Read the model definition and answer for the solid it produces. Units are mm, in the model's axes. Face numbers are marked on the shaded views. A direction names the side the tool comes from. Round coordinates to 2 decimals unless told otherwise and drop trailing zeros. Loops run counter-clockwise (first coordinate to the right, second up) from the corner with the lowest first, then second, coordinate; pieces in that order, holes last. Notation, with made-up numbers: (7.5, 1) -> (11.5, 1) arc R5 ccw to (11.5, 8) -> close; hole circle Ø6 at (61, -38.75). An arc over 180 degrees is marked (long way). Put each result on its own line as item: value.
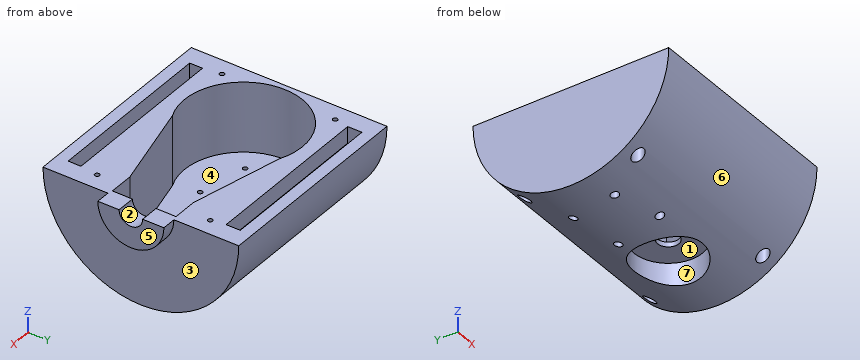
from build123d import *

# Parameters (mm, degrees)
BOSS_EXTRUDE2_DEPTH = 87
CUT_EXTRUDE1_DEPTH  = 29.5
SKETCH3_R           = 4.5
SKETCH3_R_2         = 1
CUT_EXTRUDE2_DEPTH  = 130.771336418
SKETCH4_R           = 14.5
SKETCH4_R_2         = 1.7
CUT_EXTRUDE3_DEPTH  = 10
BOSS_EXTRUDE3_START = 2
BOSS_EXTRUDE3_DEPTH = 2
BOSS_EXTRUDE4_START = 6
BOSS_EXTRUDE4_DEPTH = 6
SKETCH7_W           = 73
SKETCH7_H           = 6
SKETCH7_H_2         = 5.446782016
CUT_EXTRUDE4_DEPTH  = 7
SKETCH8_R           = 1
CUT_EXTRUDE5_DEPTH  = 136.438914135
SKETCH9_R           = 2.5
CUT_EXTRUDE6_DEPTH  = 32


with BuildPart() as part:
    # Sketch1 → Boss-Extrude2 (new body)
    with BuildSketch(Plane(origin=(89.94373008, 0, 0), x_dir=(0, 0, -1), z_dir=(1, 0, 0))):
        with BuildLine():
            Line((-104.016306216, 83.836001664), (-104.016306216, 0.836001664))
            ThreePointArc((-104.016306216, 0.836001664), (-62.516306216, 42.336001664), (-104.016306216, 83.836001664))
        make_face()
    extrude(amount=-BOSS_EXTRUDE2_DEPTH)

    # Sketch2 → Cut-Extrude1 (cut)
    with BuildSketch(Plane.XY.offset(104.016306216)):
        with BuildLine():
            Line((89.94373008, 55.836001595), (79.445092487, 55.836001664))
            Line((79.445092487, 55.836001664), (40.551337791, 64.805487997))
            ThreePointArc((40.551337791, 64.805487997), (5.067466824, 42.109927869), (40.551337791, 19.414367741))
            Line((40.551337791, 19.414367741), (79.445092487, 28.836001664))
            Line((79.445092487, 28.836001664), (89.94373008, 28.836001664))
            Line((89.94373008, 28.836001664), (89.94373008, 55.836001595))
        make_face()
    extrude(amount=-CUT_EXTRUDE1_DEPTH, mode=Mode.SUBTRACT)

    # Sketch3 → Cut-Extrude2 (cut, through all)
    with BuildSketch(Plane(origin=(0, 0, 62.516306216), x_dir=(-1, 0, 0), z_dir=(0, 0, -1))):
        with Locations(Location((-61.067466824, 42.109927869, 0), (0, 0, 90))):
            Circle(SKETCH3_R)
        with Locations(Location((-42.657418818, 50.264258545, 0), (0, 0, 90))):
            Circle(SKETCH3_R_2)
        with Locations(Location((-21.913136148, 54.699879864, 0), (0, 0, 90))):
            Circle(SKETCH3_R_2)
        with Locations(Location((-38.2217975, 29.519975875, 0), (0, 0, 90))):
            Circle(SKETCH3_R_2)
        with Locations(Location((-17.477514829, 33.955597193, 0), (0, 0, 90))):
            Circle(SKETCH3_R_2)
    extrude(amount=-CUT_EXTRUDE2_DEPTH, mode=Mode.SUBTRACT)

    # Sketch4 → Cut-Extrude3 (cut)
    with BuildSketch(Plane(origin=(0, 0, 62.516306216), x_dir=(-1, 0, 0), z_dir=(0, 0, -1))):
        with Locations(Location((-61.067466824, 42.109927869, 0), (0, 0, 90))):
            Circle(SKETCH4_R)
        with Locations(Location((-42.657418818, 50.264258545, 0), (0, 0, 90))):
            Circle(SKETCH4_R_2)
        with Locations(Location((-21.913136148, 54.699879864, 0), (0, 0, 90))):
            Circle(SKETCH4_R_2)
        with Locations(Location((-38.2217975, 29.519975875, 0), (0, 0, 90))):
            Circle(SKETCH4_R_2)
        with Locations(Location((-17.477514829, 33.955597193, 0), (0, 0, 90))):
            Circle(SKETCH4_R_2)
    extrude(amount=-CUT_EXTRUDE3_DEPTH, mode=Mode.SUBTRACT)

    # Sketch5 → Boss-Extrude3 (add)
    with BuildSketch(Plane(origin=(89.94373008, 0, 0), x_dir=(0, 0, -1), z_dir=(1, 0, 0)).offset(BOSS_EXTRUDE3_START)):
        with BuildLine():
            Line((-104.016306216, 55.836001595), (-104.016306216, 47.336001664))
            ThreePointArc((-104.016306216, 47.336001664), (-99.016306216, 42.336001664), (-104.016306216, 37.336001664))
            Line((-104.016306216, 37.336001664), (-104.016306216, 28.836001664))
            Line((-104.016306216, 28.836001664), (-104.016306216, 0.836001664))
            ThreePointArc((-104.016306216, 0.836001664), (-62.516306216, 42.336001664), (-104.016306216, 83.836001664))
            Line((-104.016306216, 83.836001664), (-104.016306216, 55.836001595))
        make_face()
    extrude(amount=-BOSS_EXTRUDE3_DEPTH)

    # Sketch6 → Boss-Extrude4 (add)
    with BuildSketch(Plane(origin=(91.94373008, 0, 0), x_dir=(0, 0, -1), z_dir=(1, 0, 0)).offset(BOSS_EXTRUDE4_START)):
        with BuildLine():
            Line((-104.016306216, 56.336001664), (-104.016306216, 47.336001664))
            ThreePointArc((-104.016306216, 47.336001664), (-99.016306216, 42.336001664), (-104.016306216, 37.336001664))
            Line((-104.016306216, 37.336001664), (-104.016306216, 28.336001664))
            ThreePointArc((-104.016306216, 28.336001664), (-90.016306216, 42.336001664), (-104.016306216, 56.336001664))
        make_face()
    extrude(amount=-BOSS_EXTRUDE4_DEPTH)

    # Sketch7 → Cut-Extrude4 (cut)
    with BuildSketch(Plane.XY.offset(104.016306216)):
        with Locations((47.44373008, 75.836001664)):
            Rectangle(SKETCH7_W, SKETCH7_H)
        with Locations((47.44373008, 8.559392672)):
            Rectangle(SKETCH7_W, SKETCH7_H_2)
    extrude(amount=-CUT_EXTRUDE4_DEPTH, mode=Mode.SUBTRACT)

    # Sketch8 → Cut-Extrude5 (cut, through all)
    with BuildSketch(Plane(origin=(0, 0, 62.516306216), x_dir=(-1, 0, 0), z_dir=(0, 0, -1))):
        with Locations(Location((-84.94373008, 66.836001664, 0), (0, 0, 90))):
            Circle(SKETCH8_R)
        with Locations(Location((-84.94373008, 18.836001664, 0), (0, 0, 90))):
            Circle(SKETCH8_R)
        with Locations(Location((-9.94373008, 66.836001664, 0), (0, 0, 90))):
            Circle(SKETCH8_R)
        with Locations(Location((-9.94373008, 18.836001664, 0), (0, 0, 90))):
            Circle(SKETCH8_R)
    extrude(amount=-CUT_EXTRUDE5_DEPTH, mode=Mode.SUBTRACT)

    # Sketch9 → Cut-Extrude6 (cut)
    with BuildSketch(Plane(origin=(0, 0, 62.516306216), x_dir=(-1, 0, 0), z_dir=(0, 0, -1))):
        with Locations(Location((-84.94373008, 66.836001664, 0), (0, 0, 90))):
            Circle(SKETCH9_R)
        with Locations(Location((-84.94373008, 18.836001664, 0), (0, 0, 90))):
            Circle(SKETCH9_R)
        with Locations(Location((-9.94373008, 66.836001664, 0), (0, 0, 90))):
            Circle(SKETCH9_R)
        with Locations(Location((-9.94373008, 18.836001664, 0), (0, 0, 90))):
            Circle(SKETCH9_R)
    extrude(amount=-CUT_EXTRUDE6_DEPTH, mode=Mode.SUBTRACT)


solid = part.part
Item 1: The part is cut by section A-A (z = 88). Determine the outline of the cut face in (x, y), then the cut area to 3 significant figures.
Derived:
outline: (2.94, 4.05) -> (91.94, 4.05) -> (91.94, 80.62) -> (2.94, 80.62) -> close; hole circle Ø5 at (9.94, 18.84); hole circle Ø5 at (9.94, 66.84); hole (40.55, 19.41) -> (79.45, 28.84) -> (89.94, 28.84) -> (89.94, 55.84) -> (79.45, 55.84) -> (40.55, 64.81) arc R25 ccw (long way) to start; hole circle Ø5 at (84.94, 18.84); hole circle Ø5 at (84.94, 66.84)
area: 3,550 mm^2
Item 2: Which of the six approach directions +Z, -Z, +X, -X, +Y, -Y give full straight-line access (tool end or side, diameter ignored) to the marked faces 1, 2, 3 and 4?
Derived:
face 1: -Z
face 2: +Z, +X
face 3: -Z, +X
face 4: +Z
Item 3: The part is cut by section C-C (x = 63.5). Determine the outline of the cut face in (y, z), then the cut area to 3 significant figures.
Derived:
outline: (0.84, 104.02) arc R41.5 ccw to (27.82, 65.14) -> (27.82, 72.52) -> (38.32, 72.52) -> (38.32, 74.52) -> (24.97, 74.52) -> (24.97, 104.02) -> (11.28, 104.02) -> (11.28, 97.02) -> (5.84, 97.02) -> (5.84, 104.02) -> close; (45.9, 72.52) -> (56.4, 72.52) -> (56.4, 64.97) arc R41.5 ccw to (83.84, 104.02) -> (78.84, 104.02) -> (78.84, 97.02) -> (72.84, 97.02) -> (72.84, 104.02) -> (59.51, 104.02) -> (59.51, 74.52) -> (45.9, 74.52) -> close
area: 1,330 mm^2
Item 4: For a pull along Y with two mould halves and no side action, classify the marked faces 5, 6 and 7 as pulls with the +Y half, pulls with the -Y half, needs draft (parallel to the pull), parting line crosses it, or undercut.
Derived:
face 5: needs draft
face 6: parting line crosses it
face 7: undercut
Item 5: Flat-ended cylindrical pins translate along their axes: pin 1 Ø2 at (x, z) = (72, 79.5) entering from -Y; pin 2 Ø10 at (x, y) = (54.5, 38.5) entering from -Z; pin 3 Ø4 at (x, y) = (42.66, 50.26) entering from -Z. Find the tip coordinate at first contact, or state that the pin passes through.
Derived:
pin 1: stops at y = 8.14
pin 2: stops at z = 72.52
pin 3: stops at z = 62.94
Item 6: The part is cut by section D-D (x = 74.5). Determine the outline of the cut face in (y, z).
Derived:
outline: (0.84, 104.02) arc R41.5 ccw to (36.65, 62.91) -> (36.65, 72.52) -> (47.57, 72.52) -> (47.57, 62.85) arc R41.5 ccw to (83.84, 104.02) -> (78.84, 104.02) -> (78.84, 97.02) -> (72.84, 97.02) -> (72.84, 104.02) -> (56.98, 104.02) -> (56.98, 74.52) -> (27.64, 74.52) -> (27.64, 104.02) -> (11.28, 104.02) -> (11.28, 97.02) -> (5.84, 97.02) -> (5.84, 104.02) -> close
Item 7: The part is cut by section B-B (y = 45). Determine the outline of the cut face in (x, z).
Derived:
outline: (2.94, 62.6) -> (46.86, 62.6) -> (46.86, 72.52) -> (57.62, 72.52) -> (57.62, 74.52) -> (5.24, 74.52) -> (5.24, 104.02) -> (2.94, 104.02) -> close; (64.52, 72.52) -> (75.28, 72.52) -> (75.28, 62.6) -> (91.94, 62.6) -> (91.94, 90.27) -> (97.94, 90.27) -> (97.94, 99.79) -> (89.94, 99.79) -> (89.94, 74.52) -> (64.52, 74.52) -> close
Item 8: Find the intervals of material crossed by line 1 along X through (y, z) = (31.5, 85.5); line 2 along Y through (x, z) = (14.5, 101.5); line 3 along X through (y, z) = (36, 85.5), in increasing order.
Derived:
line 1: x = 2.94 to 7.43, 89.94 to 91.94
line 2: y = 0.91 to 5.84, 11.28 to 22.55, 61.67 to 72.84, 78.84 to 83.76
line 3: x = 2.94 to 5.83, 89.94 to 91.94
